Part model, mm, in its own coordinate system. A direction names the side the tool comes from. Round coordinates to 2 decimals unless told otherwise and drop trailing zeros. Loops run counter-clockwise (first coordinate to the right, second up) from the corner with the lowest first, then second, coordinate; pieces in that order, holes last. Notation, with made-up numbers: M -38.75,45.5 L -0.75,45.5 A28 cw -0.75,67.5 Z; hole C 2,-9.5 d7. An arc over 180 degrees is marked long. Answer as CSV lines item,"result". Start each with the question number.
Item 1: Which spindle directions (+Z, -Z, +X, -X, +Y, -Y) get a long thin tool onto all of the face, cutting with end or side? Do faces 1 (the flat face through (68, -6, 51)), 2 (the flat face through (66.5, 16, 32)), 3 (the flat face through (62, -5, 1)). Say none if no direction does.
Item 2: Band-saw the part on C-C (y = -15). Give the cut face in (x, z).
Item 3: Drop flat-ended pins along their axis: pin 1 Ø2.5 at (x, y) = (7.12, 43.54) entering from +Z; pin 2 Ø4 at (y, z) = (0, 46) entering from +X; pin 3 Ø5 at (x, y) = (41.5, 20.5) entering from +Z; pin 4 Ø2.5 at (x, z) = (68.5, 44) entering from -Y. Give the stop position or say it passes through.
Item 4: Band-saw the part on B-B (z = 53). Give the cut face in (x, y), and give its area (3 significant figures).
Item 5: Band-saw the part on D-D (z = 36.5). Give the cut face in (x, y).
Item 6: Band-saw the part on A-A (y = -5). Count the separate pieces of the cut face and the enclosed holes in it, and give its area (3 significant figures).
Item 7: Mould opens along Y. For faces 4 (the cylindrical face through (-34.792, -8.549, 1.479)), 5 (the cylindrical face through (68, -20.07, 30.42)) say: pulls with the +Y half, pulls with the -Y half, needs draft (parallel to the pull), parting line crosses it, or undercut.
Item 8: Wall check: line 1 (X direction, y = 0, z = 2); line 2 (Y direction, x = -26.7, z = 1.8); line 3 (Y direction, x = -0.5, z = 40.5). Give the ranges that are in metal, low to high.
```python
from build123d import *

# Parameters (mm, degrees)
F0_R     = 2
F0_R_2   = 11
F0_W     = 16.8
F0_H     = 13.5
F1_DEPTH = 3
F2_DEPTH = 60
F3_W     = 14
F3_H     = 16
F4_DEPTH = 69.501
F5_R     = 2
F6_R     = 5


with BuildPart() as f1:
    # F0 (on Top) → F1 (new body)
    with BuildSketch(Plane.XY):
        Polygon((-66.5, -18.5), (66.5, -18.5), (66.5, 15.5), (66.5, 50.5), (-66.5, 50.5), (-66.5, 15.5), align=None)
        with Locations((-60.55, -9.15)):
            Circle(F0_R, mode=Mode.SUBTRACT)
        with Locations((-36.7, -9.15)):
            Circle(F0_R, mode=Mode.SUBTRACT)
        with Locations((-12.85, -9.15)):
            Circle(F0_R, mode=Mode.SUBTRACT)
        with Locations((-50.55, 0.85)):
            Circle(F0_R_2, mode=Mode.SUBTRACT)
        with Locations((-40.55, 10.85)):
            Circle(F0_R, mode=Mode.SUBTRACT)
        with Locations((-26.7, 0.85)):
            Circle(F0_R_2, mode=Mode.SUBTRACT)
        with Locations((-2.85, 0.85)):
            Circle(F0_R_2, mode=Mode.SUBTRACT)
        with Locations((-16.7, 10.85)):
            Circle(F0_R, mode=Mode.SUBTRACT)
        with Locations((11, -9.15)):
            Circle(F0_R, mode=Mode.SUBTRACT)
        with Locations((53.6, -4.75)):
            Rectangle(F0_W, F0_H, mode=Mode.SUBTRACT)
        with Locations((21, 0.85)):
            Circle(F0_R_2, mode=Mode.SUBTRACT)
        with Locations((7.15, 10.85)):
            Circle(F0_R, mode=Mode.SUBTRACT)
        with Locations((31, 10.85)):
            Circle(F0_R, mode=Mode.SUBTRACT)
        with Locations((-60.577411, 23.536334)):
            Circle(F0_R, mode=Mode.SUBTRACT)
        with Locations((-36.727411, 23.536334)):
            Circle(F0_R, mode=Mode.SUBTRACT)
        with Locations((-50.577411, 33.536334)):
            Circle(F0_R_2, mode=Mode.SUBTRACT)
        with Locations((-12.877411, 23.536334)):
            Circle(F0_R, mode=Mode.SUBTRACT)
        with Locations((-26.727411, 33.536334)):
            Circle(F0_R_2, mode=Mode.SUBTRACT)
        with Locations((-2.877411, 33.536334)):
            Circle(F0_R_2, mode=Mode.SUBTRACT)
        with Locations((-40.577411, 43.536334)):
            Circle(F0_R, mode=Mode.SUBTRACT)
        with Locations((-16.727411, 43.536334)):
            Circle(F0_R, mode=Mode.SUBTRACT)
        with Locations((10.972589, 23.536334)):
            Circle(F0_R, mode=Mode.SUBTRACT)
        with Locations((20.972589, 33.536334)):
            Circle(F0_R_2, mode=Mode.SUBTRACT)
        with Locations((53.572589, 26.986334)):
            Rectangle(F0_W, F0_H, mode=Mode.SUBTRACT)
        with Locations((7.122589, 43.536334)):
            Circle(F0_R, mode=Mode.SUBTRACT)
        with Locations((30.972589, 43.536334)):
            Circle(F0_R, mode=Mode.SUBTRACT)
    extrude(amount=F1_DEPTH)

    # F0 (on Top) → F2 (join)
    with BuildSketch(Plane.XY):
        Polygon((69.5, -15.5), (69.5, 15.5), (69.5, 53.5), (-69.5, 53.5), (-69.5, 15.5), (-69.5, -15.5), (-69.5, -21.5), (-63.5, -21.5), (63.5, -21.5), (69.5, -21.5), align=None)
        Polygon((66.5, 15.5), (66.5, -18.5), (-66.5, -18.5), (-66.5, 15.5), (-66.5, 50.5), (66.5, 50.5), align=None, mode=Mode.SUBTRACT)
    extrude(amount=F2_DEPTH)

    # F3 (on Right) → F4 (cut, through all)
    with BuildSketch(Plane.YZ):
        with Locations((-5.5, 43)):
            Rectangle(F3_W, F3_H)
        with Locations((27.236, 43)):
            Rectangle(F3_W, F3_H)
    extrude(amount=F4_DEPTH, mode=Mode.SUBTRACT)

    # F5
    f5_edges = [f1.edges().sort_by_distance(p)[0] for p in [
        (66.5, -18.5, 31.5),
        (-66.5, -18.5, 31.5),
        (-66.5, 50.5, 31.5),
        (66.5, 50.5, 31.5),
        (66.5, 16, 3),
        (0, 50.5, 3),
        (0, -18.5, 3),
        (-66.5, 16, 3),
    ]]
    fillet(f5_edges, radius=F5_R)

    # F6
    f6_edges = [f1.edges().sort_by_distance(p)[0] for p in [
        (69.5, -21.5, 30),
        (69.5, 53.5, 30),
        (-69.5, 53.5, 30),
        (-69.5, -21.5, 30),
    ]]
    fillet(f6_edges, radius=F6_R)


solid = f1.part
```
Answer block:
1,face 1,"+X"
1,face 2,"+Z"
1,face 3,"+Z, -Z"
2,outline,"M -69.5,0 L 69.5,0 L 69.5,60 L 66.5,60 L 66.5,5 A2 cw 64.5,3 L -64.5,3 A2 cw -66.5,5 L -66.5,60 L -69.5,60 Z"
3,pin 1,"passes through"
3,pin 2,"stops at x = 69.5"
3,pin 3,"stops at z = 3"
3,pin 4,"stops at y = -20.68"
4,outline,"M -69.5,-16.5 A5 ccw -64.5,-21.5 L 64.5,-21.5 A5 ccw 69.5,-16.5 L 69.5,48.5 A5 ccw 64.5,53.5 L -64.5,53.5 A5 ccw -69.5,48.5 Z; hole M -66.5,-16.5 A2 ccw -64.5,-18.5 L 64.5,-18.5 A2 ccw 66.5,-16.5 L 66.5,48.5 A2 ccw 64.5,50.5 L -64.5,50.5 A2 ccw -66.5,48.5 Z"
4,area,"1,230 mm^2"
5,outline,"M -69.5,-16.5 A5 ccw -64.5,-21.5 L 64.5,-21.5 A5 ccw 69.5,-16.5 L 69.5,-12.5 L 66.5,-12.5 L 66.5,-16.5 A2 cw 64.5,-18.5 L -64.5,-18.5 A2 cw -66.5,-16.5 L -66.5,48.5 A2 cw -64.5,50.5 L 64.5,50.5 A2 cw 66.5,48.5 L 66.5,34.24 L 69.5,34.24 L 69.5,48.5 A5 ccw 64.5,53.5 L -64.5,53.5 A5 ccw -69.5,48.5 Z; M 66.5,1.5 L 69.5,1.5 L 69.5,20.24 L 66.5,20.24 Z"
6,separate pieces,"7"
6,enclosed holes,"0"
6,area,"439 mm^2"
7,face 4,"undercut"
7,face 5,"pulls with the -Y half"
8,line 1,"x = -69.5 to -61.52, -39.58 to -37.67, -15.73 to -13.82, 8.12 to 10.03, 31.97 to 45.2, 62 to 69.5"
8,line 2,"y = -21.5 to -10.15, 11.85 to 22.54, 44.54 to 53.5"
8,line 3,"y = -21.5 to -18.5, 50.5 to 53.5"
